Model file for the job. Use its own axes, mm. Give positions to 0.01 mm unless a question says otherwise; leave off trailing zeros. Write each loop counter-clockwise with the first axis right and the second up, starting at its lowest first coordinate (ties: lowest second). Pieces come first, ordered by that corner, then holes.
Autodesk Inventor part; units mm, degrees
ref_plane "YZ Plane" through (0, 0, 0) normal (1, 0, 0) x (0, 1, 0)
ref_plane "XZ Plane" through (0, 0, 0) normal (0, 1, 0) x (-1, 0, 0)
ref_plane "XY Plane" through (0, 0, 0) normal (0, 0, 1) x (1, 0, 0)
sketch "Sketch1" plane through (0, 0, 0) normal (0, 0, 1) x (1, 0, 0)
  line L0 (-5, 0) -> (5, 0)
  line L1 (0, -5) -> (5, -5) construction
  line L2 (5, 5) -> (0, 5)
  arc A0 (0, 5) -> (-5, 0) centre (0, 0) ccw
  line L3 (5, 5) -> (5, 0)
  arc A1 (-5, 0) -> (0, -5) centre (0, 0) ccw construction
  line L4 (5, 0) -> (5, -5) construction
  dimension "d0" = 10
  dimension "d1" = 5
revolve "Revolution1" add sketch "Sketch1" angle 360 about axis through (-5, 0, 0) along (1, 0, 0)
sketch "Sketch2" plane through (5, 0, 0) normal (1, 0, 0) x (0, 0, -1)
  circle A0 centre (0, 1.5) radius 0.25
  circle A1 centre (0, -1.5) radius 0.25
  line L0 (0, 1.5) -> (0, -1.5) construction
  point P0 (0, 0)
  point P1 (0, 0)
  dimension "d3" = 3
  dimension "d4" = 0.5
extrude "Extrusion1" add sketch "Sketch2" along normal blind 0.5
properties part number "diffuser"
1. Probe probe 1 along Y at (x, z) = (-0.5, -0.5); probe 2 along Y at (x, z) = (0.25, 4.5); probe 3 along Z at (x, y) = (3, -3.25). List the from-to ranges inside material, lowest first.
Calculated:
probe 1: y = -4.95 to 4.95
probe 2: y = -2.18 to 2.18
probe 3: z = -3.8 to 3.8
2. Slice it at C-C, the plane x = 2. Write the cut outline in (y, z), and give its area (3 significant figures).
Calculated:
outline: circle Ø10 at (0, 0)
area: 78.5 mm2
3. Pin check, flat tips, straight feed: P1, Ø3, axis at y = -2.5, z = 0.5, coming from the +X side; P2, Ø5, axis at x = -3, z = 4, coming from the -Y side; P3, Ø4, axis at x = -2.5, y = -1.5, coming from the +Z side; P4, Ø5, axis at y = 4, z = -2.5, coming from the +X side. Stop position of each tip, or through.
Calculated:
P1: stops at x = 5.5
P2: stops at y = -4.33
P3: stops at z = 4.92
P4: stops at x = 5
4. Slice it at A-A, the plane z = 0. Write the cut outline in (x, y), and give its area (3 significant figures).
Calculated:
outline: (0, -5) - (5, -5) - (5, -1.75) - (5.5, -1.75) - (5.5, -1.25) - (5, -1.25) - (5, 1.25) - (5.5, 1.25) - (5.5, 1.75) - (5, 1.75) - (5, 5) - (0, 5) arc R5 ccw to start
area: 89.8 mm2
5. Slice it at D-D, the plane y = 1.5. Write the cut outline in (x, z), and give its area (3 significant figures).
Calculated:
outline: (0, -4.77) - (5, -4.77) - (5, -0.25) - (5.5, -0.25) - (5.5, 0.25) - (5, 0.25) - (5, 4.77) - (0, 4.77) arc R4.77 ccw to start
area: 83.7 mm2
6. Slice it at B-B, the plane y = 3. Write the cut outline in (x, z), and give its area (3 significant figures).
Calculated:
outline: (0, -4) - (5, -4) - (5, 4) - (0, 4) arc R4 ccw to start
area: 65.1 mm2
